Design review of the part built by this model. Coordinates are the model's own, in mm. A direction names the side the tool comes from. Round coordinates to 2 decimals unless told otherwise and drop trailing zeros. Order: outer loops, then holes, each group sorted by start corner. A loop starts at its lowest first (then second) coordinate and runs counter-clockwise, first axis right, second up. Notation, with made-up numbers: M -21.75,-34 L 27.25,-34 A21 ccw 27.25,-22 Z; hole C 87.5,-4 d2. An arc over 180 degrees is marked long. Write each question's results on one line, items separated by ' | '. Start each with the question number.
Item 1: Machinability: for faces 1 (the flat face through (42, 10, -1)), 2 (the flat face through (-27, 1, 1)), 3 (the flat face through (-43, 10, -1)), which of the approach directions +Z, -Z, +X, -X, +Y, -Y give a long, thin tool a straight path to every point of the face, cutting with its end or side? Answer none if there is none.
Item 2: Take a section at C-C, the plane z = -5.5. Write out the cut boundary in (x, y).
Item 3: The part is to be moulded in two halves that separate along X. For faces 4 (the flat face through (18.87, 1.52, 0.5)), 5 (the flat face through (-25, 11, 1)), 6 (the cylindrical face through (56.39, 5.07, 32.58)), 7 (the flat face through (-1, 6, 36)), say which applies: +X half, -X half, draft (parallel to the pull), parting line (faces both ways), or undercut.
Item 4: Take a section at A-A, the plane z = 26.5. Write out the cut boundary in (x, y), plus the area to 3 significant figures.
Item 5: Take a section at B-B, the plane y = 4.75. Write out the cut boundary in (x, z), plus the area to 3 significant figures.
Item 6: Clearance check with flat-ended pins moving along their axes: pin 1 (12 mm diameter, centred on x = 29.5, z = 20, fed in from -Y); pin 2 (21 mm diameter, centred on x = -6, z = -17.5, fed in from -Y); pin 3 (2.5 mm diameter, centred on y = 12, z = 8, fed in from +X); pin 4 (15.5 mm diameter, centred on x = -48, z = -24, fed in from +Y). State where each tip first meets the part, or that it passes through.
Item 7: Take a section at D-D, the plane x = 40. Write out the cut boundary in (y, z).
Item 8: Wall thickness on line 1 (X direction, y = 5.5, z = 24); line 2 (X direction, y = 6.25, z = -22); line 3 (Z direction, x = 52.5, y = 5.5): over which ranges is each line inside the solid? List them lowest first. Write a range as [from, to].
```python
from build123d import *

# Parameters (mm, degrees)
SKETCH1_W           = 120
SKETCH1_H           = 72
BOSS_EXTRUDE1_DEPTH = 10
SKETCH2_R           = 6
CUT_EXTRUDE1_DEPTH  = 71.682388188
FILLET1_R           = 12
CUT_EXTRUDE2_DEPTH  = 95.254973344
SKETCH4_W           = 50
SKETCH4_H           = 72
BOSS_EXTRUDE3_DEPTH = 3


with BuildPart() as part:
    # Sketch1 → Boss-Extrude1 (new body)
    with BuildSketch(Plane(origin=(0, 0, 0), x_dir=(1, 0, 0), z_dir=(0, 1, 0))):
        Rectangle(SKETCH1_W, SKETCH1_H)
    extrude(amount=BOSS_EXTRUDE1_DEPTH)

    # Sketch2 → Cut-Extrude1 (cut, through all)
    with BuildSketch(Plane(origin=(0, 10, 0), x_dir=(1, 0, 0), z_dir=(0, 1, 0))):
        with Locations(Location((-48, 24, 0), (0, 0, 270))):
            Circle(SKETCH2_R)
        with Locations(Location((-48, -24, 0), (0, 0, 270))):
            Circle(SKETCH2_R)
        with Locations(Location((48, -24, 0), (0, 0, 270))):
            Circle(SKETCH2_R)
        with Locations(Location((48, 24, 0), (0, 0, 270))):
            Circle(SKETCH2_R)
    extrude(amount=-CUT_EXTRUDE1_DEPTH, mode=Mode.SUBTRACT)

    # Fillet1
    fillet1_edges = [part.edges().sort_by_distance(p)[0] for p in [
        (60, 5, 36),
        (-60, 5, 36),
        (-60, 5, -36),
        (60, 5, -36),
    ]]
    fillet(fillet1_edges, radius=FILLET1_R)

    # Sketch3 → Cut-Extrude2 (cut, through all)
    with BuildSketch(Plane.XY.offset(36)):
        Polygon((-28, 0), (-25, 3), (17.388701421, 3), (20.388701421, 0), align=None)
    extrude(amount=-CUT_EXTRUDE2_DEPTH, mode=Mode.SUBTRACT)

    # Sketch4 → Boss-Extrude3 (add)
    with BuildSketch(Plane(origin=(0, 10, 0), x_dir=(1, 0, 0), z_dir=(0, 1, 0))):
        Rectangle(SKETCH4_W, SKETCH4_H)
    extrude(amount=BOSS_EXTRUDE3_DEPTH)


solid = part.part
```
Results list:
1) face 1: +Z, -Z, +X, +Y | face 2: +Z, -Z, -Y | face 3: +Z, -Z, -X, +Y
2) outline: M -60,0 L -28,0 L -25,3 L 17.39,3 L 20.39,0 L 60,0 L 60,10 L 25,10 L 25,13 L -25,13 L -25,10 L -60,10 Z
3) face 4: undercut | face 5: -X half | face 6: +X half | face 7: draft
4) outline: M -59.74,0 L -53.45,0 L -53.45,10 L -59.74,10 Z; M -42.55,0 L -28,0 L -25,3 L 17.39,3 L 20.39,0 L 42.55,0 L 42.55,10 L 25,10 L 25,13 L -25,13 L -25,10 L -42.55,10 Z; M 53.45,0 L 59.74,0 L 59.74,10 L 53.45,10 Z | area: 990 mm²
5) outline: M -60,-24 A12 ccw -48,-36 L 48,-36 A12 ccw 60,-24 L 60,24 A12 ccw 48,36 L -48,36 A12 ccw -60,24 Z; hole C -48,-24 d12; hole C -48,24 d12; hole C 48,-24 d12; hole C 48,24 d12 | area: 8,060 mm²
6) pin 1: y = 0 | pin 2: y = 3 | pin 3: x = 25 | pin 4: y = 10
7) outline: M 0,-36 L 10,-36 L 10,36 L 0,36 Z
8) line 1: [-60, -54], [-42, 42], [54, 60] | line 2: [-60, -53.66], [-42.34, 42.34], [53.66, 60] | line 3: [-35.12, -27.97], [-20.03, 20.03], [27.97, 35.12]
